from build123d import *

# Parameters (mm, degrees)
SKETCH1_R           = 31.75
SKETCH1_R_2         = 4
BOSS_EXTRUDE1_DEPTH = 1.5
CUT_EXTRUDE1_DEPTH  = 45.926328584


with BuildPart() as part:
    # Sketch1 → Boss-Extrude1 (new body)
    with BuildSketch(Plane.XY):
        Circle(SKETCH1_R)
        with Locations((5.75, 5.75)):
            Circle(SKETCH1_R_2, mode=Mode.SUBTRACT)
        with Locations((8.338190451, 15.409258263)):
            Circle(SKETCH1_R_2, mode=Mode.SUBTRACT)
        with Locations((17.997448714, 17.997448714)):
            Circle(SKETCH1_R_2, mode=Mode.SUBTRACT)
        with Locations((15.409258263, 8.338190451)):
            Circle(SKETCH1_R_2, mode=Mode.SUBTRACT)
        with Locations((25.068516526, 5.75)):
            Circle(SKETCH1_R_2, mode=Mode.SUBTRACT)
        with Locations((5.75, 25.068516526)):
            Circle(SKETCH1_R_2, mode=Mode.SUBTRACT)
        with Locations((25.068556101, -5.749960425)):
            Circle(SKETCH1_R_2, mode=Mode.SUBTRACT)
        with Locations((15.409297838, -8.338150876)):
            Circle(SKETCH1_R_2, mode=Mode.SUBTRACT)
        with Locations((17.997488289, -17.997409139)):
            Circle(SKETCH1_R_2, mode=Mode.SUBTRACT)
        with Locations((8.338230026, -15.409218688)):
            Circle(SKETCH1_R_2, mode=Mode.SUBTRACT)
        with Locations((5.750039575, -25.068476951)):
            Circle(SKETCH1_R_2, mode=Mode.SUBTRACT)
        with Locations((5.750039575, -5.749960425)):
            Circle(SKETCH1_R_2, mode=Mode.SUBTRACT)
        with Locations((-5.74992085, -25.068516526)):
            Circle(SKETCH1_R_2, mode=Mode.SUBTRACT)
        with Locations((-8.338111301, -15.409258263)):
            Circle(SKETCH1_R_2, mode=Mode.SUBTRACT)
        with Locations((-17.997369564, -17.997448714)):
            Circle(SKETCH1_R_2, mode=Mode.SUBTRACT)
        with Locations((-15.409179113, -8.338190451)):
            Circle(SKETCH1_R_2, mode=Mode.SUBTRACT)
        with Locations((-25.068437376, -5.75)):
            Circle(SKETCH1_R_2, mode=Mode.SUBTRACT)
        with Locations((-5.74992085, -5.75)):
            Circle(SKETCH1_R_2, mode=Mode.SUBTRACT)
        with Locations((-25.068476951, 5.749960425)):
            Circle(SKETCH1_R_2, mode=Mode.SUBTRACT)
        with Locations((-15.409218688, 8.338150876)):
            Circle(SKETCH1_R_2, mode=Mode.SUBTRACT)
        with Locations((-17.997409139, 17.997409139)):
            Circle(SKETCH1_R_2, mode=Mode.SUBTRACT)
        with Locations((-8.338150876, 15.409218688)):
            Circle(SKETCH1_R_2, mode=Mode.SUBTRACT)
        with Locations((-5.749960425, 25.068476951)):
            Circle(SKETCH1_R_2, mode=Mode.SUBTRACT)
        with Locations((-5.749960425, 5.749960425)):
            Circle(SKETCH1_R_2, mode=Mode.SUBTRACT)
    extrude(amount=BOSS_EXTRUDE1_DEPTH)

    # Sketch2 → Cut-Extrude1 (cut, through all)
    with BuildSketch(Plane.XY):
        with BuildLine():
            Line((-26.149880274, 18.006839302), (0, 11))
            Line((0, 11), (26.149880274, 18.006839302))
            ThreePointArc((26.149880274, 18.006839302), (0, 31.75), (-26.149880274, 18.006839302))
        make_face()
    extrude(amount=CUT_EXTRUDE1_DEPTH, mode=Mode.SUBTRACT)


solid = part.part
Geometry: final body of the model. Coordinates: model frame, mm. A direction names the side the tool comes from. Give positions to 0.01 mm unless a question says otherwise; leave off trailing zeros. Order: outer loops, then holes, each group sorted by start corner. A loop starts at its lowest first (then second) coordinate and runs counter-clockwise, first axis right, second up. Notation, with made-up numbers: (-12.5, 55.5) -> (44.5, 55.5) arc R18 cw to (44.5, 75.5) -> close; hole circle Ø5 at (61, -18.5). An arc over 180 degrees is marked (long way). Answer as a JSON object with one key per item and string values.
Q1. Section B-B (y = -3.5). Output: boundary loops of the cut face in (x, z), plus the area to 3 significant figures.
Entries:
{"outline": "(-31.56, 0) -> (-28.38, 0) -> (-28.38, 1.5) -> (-31.56, 1.5) -> close; (-21.76, 0) -> (-9.06, 0) -> (-9.06, 1.5) -> (-21.76, 1.5) -> close; (-2.44, 0) -> (2.44, 0) -> (2.44, 1.5) -> (-2.44, 1.5) -> close; (9.06, 0) -> (21.76, 0) -> (21.76, 1.5) -> (9.06, 1.5) -> close; (28.38, 0) -> (31.56, 0) -> (31.56, 1.5) -> (28.38, 1.5) -> close", "area": "55.0 mm^2"}
Q2. Draft query along X for faces 3 (the cylindrical face through (-0.966, -31.735, 0.74)), 4 (the flat face through (0, -7, 0)), 5 (the flat face through (2.76, 11.74, 0.74)). Return one class per face: released by +X, released by -X, zero draft, split by the parting line, or undercut.
Entries:
{"face 3": "split by the parting line", "face 4": "zero draft", "face 5": "undercut"}
Q3. Section C-C (z = 0.7). State how many separate pieces and enclosed holes the cut face has, plus the area to 3 significant figures.
Entries:
{"separate pieces": "1", "enclosed holes": "18", "area": "1,540 mm^2"}
Q4. Material intervals for probe 1 along X at (y, z) = (-21.5, 1.15); probe 2 along Y at (x, z) = (-16, 1.3); probe 3 along Y at (x, z) = (8, 1.25), sorted ascending.
Entries:
{"probe 1": "x = -23.36 to -19.93, -16.07 to -7.56, -3.94 to 3.94, 7.56 to 16.07, 19.93 to 23.36", "probe 2": "y = -27.42 to -21.46, -14.53 to -12.29, -4.38 to 4.38, 12.29 to 14.53", "probe 3": "y = -30.73 to -28.38, -21.76 to -19.39, -11.42 to -9.06, -2.44 to 2.44, 9.06 to 11.42"}
Q5. Section D-D (y = -27). Output: boundary loops of the cut face in (x, z).
Entries:
{"outline": "(-16.71, 0) -> (-9.25, 0) -> (-9.25, 1.5) -> (-16.71, 1.5) -> close; (-2.25, 0) -> (2.25, 0) -> (2.25, 1.5) -> (-2.25, 1.5) -> close; (9.25, 0) -> (16.71, 0) -> (16.71, 1.5) -> (9.25, 1.5) -> close"}
Q6. Access query for faces 1 (the cylindrical face through (19.225, -7.137, 0.74)), 2 (the flat face through (23.96, 17.42, 0.74)). Directions: +Z, -Z, +X, -X, +Y, -Y. A direction counts if a zero-diameter tool reaches every point of the face in a straight line with its end or side. Return the directions, or none.
Entries:
{"face 1": "+Z, -Z", "face 2": "+Z, -Z, +Y"}
Q7. Section A-A (x = -13). Output: boundary loops of the cut face in (y, z), plus the area to 3 significant figures.
Entries:
{"outline": "(-28.97, 0) -> (-11.53, 0) -> (-11.53, 1.5) -> (-28.97, 1.5) -> close; (-5.15, 0) -> (5.15, 0) -> (5.15, 1.5) -> (-5.15, 1.5) -> close; (11.53, 0) -> (14.48, 0) -> (14.48, 1.5) -> (11.53, 1.5) -> close", "area": "46.0 mm^2"}
